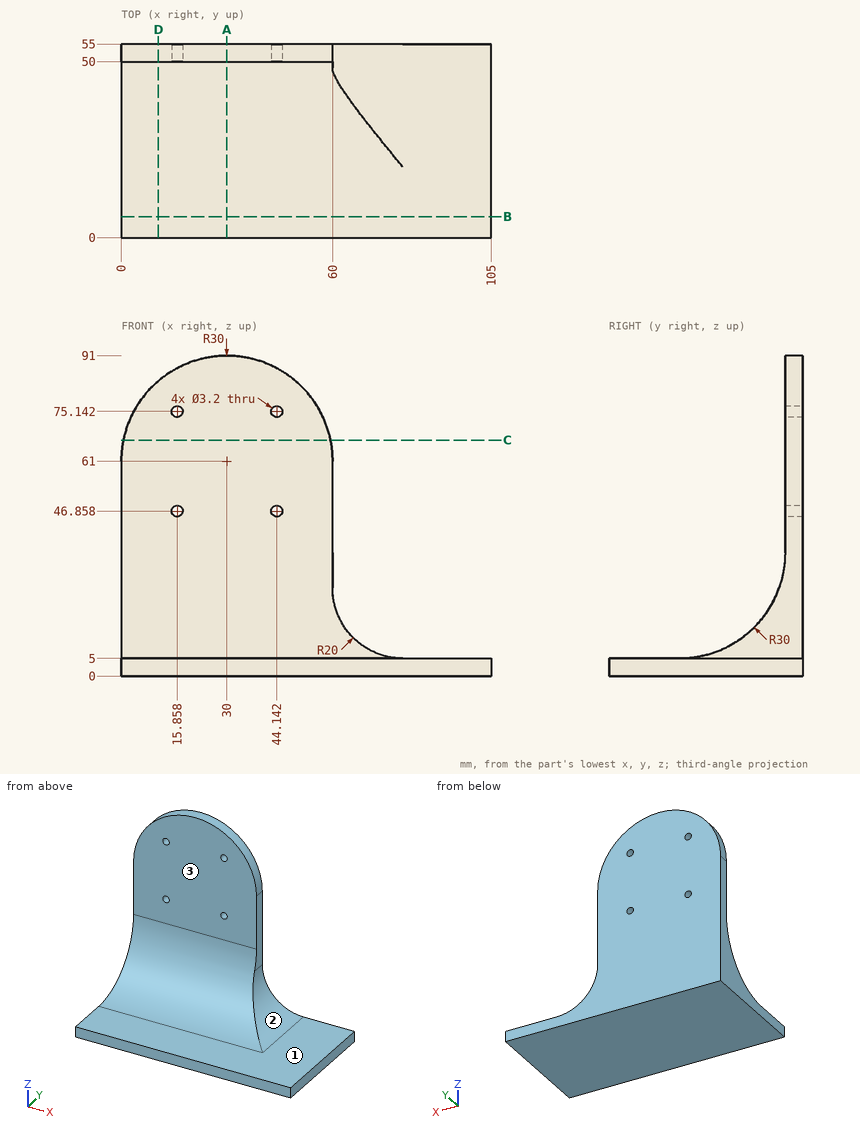
Job drawing, mm, ordinate dimensions from the low corner. One solid piece. A direction names the side the tool comes from. Give positions to 0.01 mm unless a question says otherwise; leave off trailing zeros. Order: outer loops, then holes, each group sorted by start corner. A loop starts at its lowest first (then second) coordinate and runs counter-clockwise, first axis right, second up. Notation, with made-up numbers: (65.25, 51.5) - (102.25, 51.5) arc R20 ccw to (102.25, 73.5) - close; hole circle Ø10 at (73, -14.75). An arc over 180 degrees is marked (long way). Answer in a Markdown table with one row per item.
1. Saw through at A-A, the plane x = 30. Give the cut face in (y, z).
Data:
| item | result |
|---|---|
| outline | (0, 0) - (55, 0) - (55, 91) - (50, 91) - (50, 35) arc R30 cw to (20, 5) - (0, 5) - close |
2. Saw through at D-D, the plane x = 10.5. Give the cut face in (y, z).
Data:
| item | result |
|---|---|
| outline | (0, 0) - (55, 0) - (55, 83.8) - (50, 83.8) - (50, 35) arc R30 cw to (20, 5) - (0, 5) - close |
3. Flat gauge pins, fed straight in: pin 1 (3 mm diameter, centred on x = 44.14, z = 46.86, fed in from +Y); pin 2 (5.5 mm diameter, centred on y = 50.5, z = 47, fed in from +X); pin 3 (3 mm diameter, centred on x = 88, y = 15, fed in from +Z). Where does each tip first touch, or does it go through?
Data:
| item | result |
|---|---|
| pin 1 | passes through |
| pin 2 | stops at x = 60 |
| pin 3 | stops at z = 5 |
4. Saw through at B-B, the plane y = 6. Give the cut face in (x, z), plus the area to 3 significant figures.
Data:
| item | result |
|---|---|
| outline | (0, 0) - (105, 0) - (105, 5) - (0, 5) - close |
| area | 525 mm² |
5. Tool access for the marked faces 1, 2 and 3: list every direction of +Z, -Z, +X, -X, +Y, -Y with a clear straight run to the whole face (end or side of a thin tool).
Data:
| item | result |
|---|---|
| face 1 | +Z, +X, -Y |
| face 2 | +Z, +X, +Y, -Y |
| face 3 | +Z, +X, -X, -Y |
6. Saw through at C-C, the plane z = 67. Give the cut face in (x, y).
Data:
| item | result |
|---|---|
| outline | (0.61, 50) - (59.39, 50) - (59.39, 55) - (0.61, 55) - close |
7. Probe probe 1 along Y at (x, z) = (40, 49); probe 2 along Z at (x, y) = (47, 15); probe 3 along X at (y, z) = (50.5, 38). List the from-to ranges inside material, lowest first. Write a range as [from, to].
Data:
| item | result |
|---|---|
| probe 1 | y = [50, 55] |
| probe 2 | z = [0, 5] |
| probe 3 | x = [0, 60] |
